Solid Edge part; units mm, degrees
sketch "Sketch1" plane through (0, 0, 0) normal (1, 0, 0) x (0, 1, 0)
  line L0 (-41.0882, 24.973) -> (-23.3024, 38.5623)
  line L1 (-12.9904, 36.5) -> (6.0622, 3.5)
  line L2 (1.6596, -6.8004) -> (-10.8671, -9.8574)
  line L3 (-12.0526, -10) -> (-38.0526, -10)
  line L4 (-43.0526, -5) -> (-43.0526, 21)
  arc A0 (-23.3024, 38.5623) -> (-12.9904, 36.5) centre (-19.0526, 33) cw
  arc A1 (6.0622, 3.5) -> (1.6596, -6.8004) centre (0, 0) cw
  arc A2 (-10.8671, -9.8574) -> (-12.0526, -10) centre (-12.0526, -5) cw
  arc A3 (-38.0526, -10) -> (-43.0526, -5) centre (-38.0526, -5) cw
  arc A4 (-43.0526, 21) -> (-41.0882, 24.973) centre (-38.0526, 21) cw
  circle A5 centre (-19.0526, 33) radius 3.2
  circle A6 centre (0, 0) radius 3.2
  circle A7 centre (-12.0526, -5) radius 1.7
  circle A8 centre (-12.0526, 21) radius 1.7
  circle A9 centre (-38.0526, 21) radius 1.7
  circle A10 centre (-38.0526, -5) radius 1.7
  circle A11 centre (-25.0526, 8) radius 13
extrude "Protrusion1" add sketch "Sketch1" against normal blind 9
sketch "Sketch2" plane through (0, -18.0263, 15) normal (1, 0, 0) x (0, 1, 0)
  circle A0 centre (15.5263, 7.5) radius 1.7
  arc A1 (24.0885, -11.5) -> (24.0604, -18.5481) centre (18.0263, -15) cw
  line L0 (24.0604, -18.5481) -> (32.5912, -4.04)
  line L1 (5.0359, 21.5) -> (31.3808, 1.7077)
  line L2 (5.0359, 21.5) -> (24.0885, -11.5)
  arc A2 (32.5912, -4.04) -> (31.3808, 1.7077) centre (28.0263, -2) ccw
  circle A3 centre (28.0263, -2) radius 1.7
extrude "ExtrudedProtrusion_2" add sketch "Sketch2" against normal blind 9
sketch "Sketch3" plane through (0, -14.0263, 15) normal (1, 0, 0) x (0, 1, 0)
  line L0 (6.6856, 1.1307) -> (19.1856, -8.3693)
  line L1 (25.1318, -9.9232) -> (28.5912, -4.04)
  arc A0 (28.5912, -4.04) -> (27.3808, 1.7077) centre (24.0263, -2) ccw
  line L2 (27.3808, 1.7077) -> (9.4039, 15.2133)
  arc A1 (9.4039, 15.2133) -> (6.6856, 1.1307) centre (11.5263, 7.5) ccw
  arc A2 (19.1856, -8.3693) -> (25.1318, -9.9232) centre (24.0263, -2) ccw
  circle A3 centre (11.5263, 7.5) radius 1.7
  circle A4 centre (24.0263, -2) radius 1.7
extrude "ExtrudedProtrusion_4" add sketch "Sketch3" along normal blind 4
sketch "Sketch4" plane through (0, -15.9735, 15) normal (1, 0, 0) x (0, 0, 1)
  circle A0 centre (6, -3.9209) radius 4
extrude "Cutout1" cut sketch "Sketch4" along normal through all
sketch "Sketch5" plane through (-9, -14.0263, 15) normal (-1, 0, 0) x (0, -1, 0)
  line L0 (-23.3897, 4.7061) -> (-5.4027, 18.2193)
  line L1 (-18.3897, 18.2193) -> (-5.4027, 18.2193)
  line L2 (-23.3897, 13.2193) -> (-23.3897, 4.7061)
  arc A0 (-18.3897, 18.2193) -> (-23.3897, 13.2193) centre (-18.3897, 13.2193) ccw
  circle A1 centre (-18.3897, 13.2193) radius 1.7
extrude "ExtrudedProtrusion_5" add sketch "Sketch5" against normal blind 5
properties material "ABS Plastic, high impact"
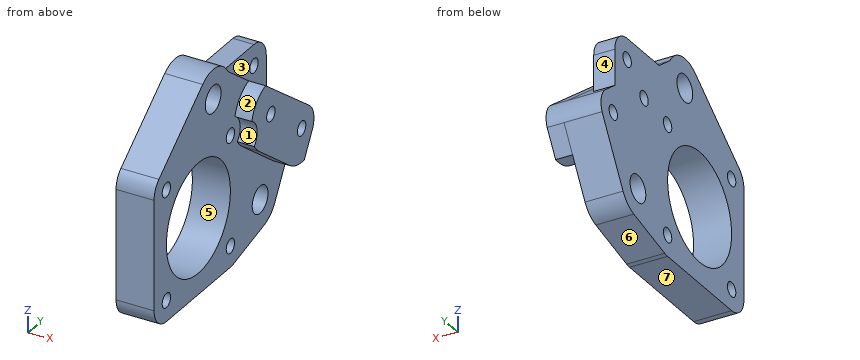
Geometry check sheet. Reference: the model listing, model coordinates, mm. Face numbers are marked on the shaded views. A direction names the side the tool comes from. Round coordinates to 2 decimals unless told otherwise and drop trailing zeros. Loops run counter-clockwise (first coordinate to the right, second up) from the corner with the lowest first, then second, coordinate; pieces in that order, holes last. Notation, with made-up numbers: (59.25, 18) -> (71.25, 18) arc R24 ccw to (71.25, 51) -> close; hole circle Ø11 at (51, 33.5). An arc over 180 degrees is marked (long way). Answer as a JSON object with one key per item and string values. Group by question number.
Item 1: Cross-section at C-C, the plane x = -6.25. Count the separate pieces of the cut face and the enclosed holes in it, plus the area to 3 significant figures.
Item 2: Cross-section at B-B, the plane z = 8. Record the cut outline in (x, y).
Item 3: Cross-section at A-A, the plane y = 10. Record the cut outline in (x, z).
Item 4: Set-up check for the marked faces 1, 2, 3 and 4: record each of +Z, -Z, +X, -X, +Y, -Y from which the full face is reachable in a straight line by a thin tool's end or side.
Item 5: Depth check by flat-ended pin: pin 1 Ø25 at (y, z) = (-10.5, 24.5) entering from +X; pin 2 Ø2 at (x, z) = (1.5, 7) entering from -Y; pin 3 Ø5.5 at (x, z) = (-7, 24.5) entering from +Y; pin 4 Ø3 at (x, z) = (-7, 31) entering from +Y. Enter the tip coordinate at first touch or a pass-through.
Item 6: Thickness scan on line 1 along Y through (x, z) = (-8.25, -1); line 2 along Z through (x, y) = (-7.5, -16.5); line 3 along X through (y, z) = (-23, 25). Record the ranges inside material, lowest first.
Item 7: Release check for a two-part mould opening along Y. For the marked faces 5, 6 and 7 record: pulls with the +Y half, pulls with the -Y half, needs draft (parallel to the pull), parting line crosses it, or undercut.
Item 8: Cross-section at D-D, the plane z = 0. Record the cut outline in (x, y), plus the area to 3 significant figures.
Determined:
{
 "1": {"separate pieces": "1", "enclosed holes": "10", "area": "1,610 mm²"},
 "2": {"outline": "(-9, -43.05) -> (0, -43.05) -> (0, -38.05) -> (-9, -38.05) -> close; (-9, -12.05) -> (0, -12.05) -> (0, 3.36) -> (4, 3.36) -> (4, 12.82) -> (-9, 12.82) -> close"},
 "3": {"outline": "(-9, 3.2) -> (0, 3.2) -> (0, 5) -> (4, 5) -> (4, 11.3) -> (-9, 11.3) -> close; (-9, 14.7) -> (4, 14.7) -> (4, 19.23) -> (-9, 19.23) -> close"},
 "4": {"face 1": "+X, -Y", "face 2": "+Z, +X, -Y", "face 3": "+Z, +X, +Y", "face 4": "+Z, +X, -X, +Y"},
 "5": {"pin 1": "stops at x = 4", "pin 2": "stops at y = 3.36", "pin 3": "stops at y = 9.36", "pin 4": "stops at y = 9.2"},
 "6": {"line 1": "y = -43.05 to -34.43, -15.67 to -3.04, 3.04 to 7.53", "line 2": "z = -10 to -1.79, 17.79 to 31.07, 34.93 to 39.52", "line 3": "x = -9 to 0"},
 "7": {"face 5": "undercut", "face 6": "pulls with the +Y half", "face 7": "needs draft"},
 "8": {"outline": "(-9, -43.05) -> (0, -43.05) -> (0, -35.3) -> (-9, -35.3) -> close; (-9, -14.81) -> (0, -14.81) -> (0, -3.2) -> (-9, -3.2) -> close; (-9, 3.2) -> (0, 3.2) -> (0, 8.12) -> (-9, 8.12) -> close", "area": "219 mm²"}
}
